Autodesk Inventor part; units mm, degrees
ref_plane "YZ Plane" through (0, 0, 0) normal (1, 0, 0) x (0, 1, 0)
ref_plane "XZ Plane" through (0, 0, 0) normal (0, 1, 0) x (-1, 0, 0)
ref_plane "XY Plane" through (0, 0, 0) normal (0, 0, 1) x (1, 0, 0)
sketch "Sketch1" plane through (0, 0, 0) normal (1, 0, 0) x (0, 1, 0)
  line L0 (0, 0) -> (-40.0558, 0)
  line L1 (-40.0558, 0) -> (-40.0558, -6.35)
  line L2 (-40.0558, -6.35) -> (0, -6.35)
  line L3 (0, -6.35) -> (0, 0)
  line L4 (-23.495, -6.35) -> (-34.0019, 4.1569)
  line L5 (-34.0019, 4.1569) -> (-42.2823, -4.1235)
  line L6 (-42.2823, -4.1235) -> (-31.7754, -14.6304)
  line L7 (-31.7754, -14.6304) -> (-23.495, -6.35)
  line L8 (-23.495, -6.35) -> (-8.636, -6.35) construction
  line L9 (-23.495, -6.35) -> (0, -6.35) construction
  dimension "d0" = 40.0558
  dimension "d2" = 6.35
  dimension "d3" = 14.859
  dimension "d4" = 135
  dimension "d6" = 23.495
extrude "Extrusion1" add sketch "Sketch1" along normal blind 26.3652
sketch "Sketch2" plane through (26.3652, 0, 0) normal (1, 0, 0) x (0, 0, -1)
  line L0 (6.35, -23.495) -> (6.35, 0)
  line L1 (6.35, 0) -> (0, 0)
  line L2 (0, 0) -> (0, -29.845)
  line L3 (14.6304, -31.7754) -> (6.35, -23.495)
  line L4 (6.35, -23.495) -> (0, -29.845)
  line L5 (0, -29.845) -> (0, 0)
  line L6 (0, 0) -> (6.35, 0)
  line L7 (6.35, 0) -> (6.35, -23.495)
extrude "Extrusion2" cut sketch "Sketch2" against normal blind 16.2052
sketch "Sketch5" plane through (0, 0, 0) normal (-1, 0, 0) x (0, 0, 1)
  line L0 (-4.1235, -42.2823) -> (-14.6304, -31.7754)
  line L1 (-6.35, -23.495) -> (-6.35, 0)
  line L2 (-6.35, -23.495) -> (-6.35, -40.0558)
  line L3 (-6.35, -40.0558) -> (-14.6304, -31.7754)
  line L4 (-14.6304, -31.7754) -> (-6.35, -23.495)
extrude "Extrusion5" cut sketch "Sketch5" against normal blind 12.7
sketch "Sketch6" plane through (26.3652, -23.495, -6.35) normal (0, 0.7071, -0.7071) x (-1, 0, 0)
  line L0 (13.6652, -11.7103) -> (0, -11.7103)
  circle A0 centre (6.8326, -5.8551) radius 4.5085
  line L1 (13.6652, 0) -> (0, 0)
  line L2 (0, -11.7103) -> (0, 0)
  line L3 (6.8326, -5.8551) -> (6.8326, 0) construction
  line L4 (6.8326, -5.8551) -> (6.8326, -11.7103) construction
  point P0 (26.3652, 21.1036)
  dimension "d24" = 9.017
extrude "Extrusion6" cut sketch "Sketch6" against normal blind 25.4
sketch "Sketch7" plane through (0, 0, 0) normal (-1, 0, 0) x (0, 0, 1)
  line L0 (-6.35, 0) -> (-6.35, -40.0558)
  line L1 (-6.35, 0) -> (0, 0)
  circle A0 centre (-7.62, -34.9758) radius 2.54
  line L2 (-7.62, -34.9758) -> (-6.35, -34.9758) construction
  line L3 (-6.35, -34.9758) -> (-6.35, -40.0558) construction
  line L4 (-6.35, 0) -> (-6.35, -5.08) construction
  line L5 (-6.35, -5.08) -> (-7.62, -5.08) construction
  circle A1 centre (-7.62, -5.08) radius 2.54
  dimension "d27" = 1.27
  dimension "d29" = 5.08
  dimension "d30" = 5.08
  dimension "d31" = 5.08
  dimension "d32" = 1.27
  dimension "d33" = 5.08
extrude "Extrusion7" add sketch "Sketch7" against normal blind 6.35
sketch "Sketch8" plane through (0, 0, 0) normal (-1, 0, 0) x (0, 0, 1)
  line L0 (0, -29.845) -> (4.1569, -34.0019)
  line L1 (0, 0) -> (0, -29.845)
  line L2 (4.1569, -34.0019) -> (-4.1235, -42.2823)
  line L3 (-6.35, -7.2797) -> (-6.35, -32.7761)
  line L4 (4.1569, -34.0019) -> (4.1569, -26.3819)
  line L5 (4.1569, -26.3819) -> (0, -22.225)
  line L6 (0, -22.225) -> (0, -29.845)
  line L7 (4.1569, -34.0019) -> (0, -29.845)
  dimension "d42" = 7.62
extrude "Extrusion8" add sketch "Sketch8" against normal blind 12.1412
ref_plane "Work Plane1" through (12.1412, -6.35, -6.35) normal (1, 0, 0) x (0, 0, -1)
sketch "Sketch9" plane through (12.1412, -6.35, -6.35) normal (1, 0, 0) x (0, 0, -1)
  line L0 (-10.5069, 6.35) -> (-10.5069, -29.5569)
  line L1 (-6.35, -25.4) -> (-10.5069, -29.5569)
  line L2 (-6.35, -25.4) -> (-6.35, 0)
  circle A0 centre (-8.4284, -20.4934) radius 1.5875
  line L3 (-6.35, -20.4934) -> (-10.5069, -20.4934) construction
  line L4 (-8.4284, -20.4934) -> (-8.4284, -27.4784) construction
  point P0 (-6.35, 6.35)
  dimension "d38" = 3.175
  dimension "d39" = 6.985
extrude "Extrusion9" add sketch "Sketch9" along normal blind 2.54
sketch "Sketch10" plane through (26.3652, 0, 0) normal (1, 0, 0) x (0, 0, -1)
  line L0 (0, -40.0558) -> (1.897, -40.0558)
  line L1 (14.6304, -31.7754) -> (6.35, -23.495)
  line L2 (0, -38.1254) -> (1.897, -40.0558)
  line L3 (1.897, -40.0558) -> (0, -40.0558)
  line L4 (0, -38.1254) -> (0, -40.0558)
  line L5 (0, -38.1254) -> (1.897, -40.0558)
  point P0 (0, 0)
  dimension "d43" = 0.5
extrude "Extrusion10" cut sketch "Sketch10" against normal blind 38.1
sketch "Sketch11" plane through (14.6812, -26.8434, 2.0784) normal (1, 0, 0) x (0, 0, -1)
  circle A0 centre (0, 0) radius 1.5875
  circle A1 centre (0, 0) radius 1.5875
  line L0 (-1.5875, 0) -> (1.5875, 0)
  line L1 (1.5875, 0) -> (1.5875, -2.159)
  line L2 (1.5875, -2.159) -> (-1.5875, -2.159)
  line L3 (-1.5875, -2.159) -> (-1.5875, 0)
  point P0 (2.0784, 26.8434)
  dimension "d46" = 2.159
extrude "Extrusion11" add sketch "Sketch11" along normal blind 2.54
sketch "Sketch14" plane through (12.1412, -6.35, -6.35) normal (1, 0, 0) x (0, 0, -1)
  line L0 (-6.8465, -10.2985) -> (-15.1263, -2.0187)
  line L1 (8.2804, -25.4254) -> (0, -17.145)
  line L2 (-15.1263, -2.0187) -> (-25.6332, -12.5256)
  line L3 (-25.6332, -12.5256) -> (-17.3534, -20.8054)
  line L4 (-17.3534, -20.8054) -> (-6.8465, -10.2985)
  point P0 (-6.35, 6.35)
  dimension "d60" = 11.7094
  dimension "d61" = 14.859
extrude "Extrusion14" add sketch "Sketch14" along normal blind 13.6652
sketch "Sketch15" plane through (12.1412, -6.35, -6.35) normal (-1, 0, 0) x (0, 0, 1)
  line L0 (6.8465, -10.2985) -> (15.1263, -2.0187)
  line L1 (25.6332, -12.5256) -> (17.3534, -20.8054)
  line L2 (15.1263, -2.0187) -> (25.6332, -12.5256)
  line L3 (25.6332, -12.5256) -> (17.3534, -20.8054)
  line L4 (6.8465, -10.2985) -> (17.3534, -20.8054)
  line L5 (6.8465, -10.2985) -> (15.1263, -2.0187)
  point P0 (6.35, 6.35)
extrude "Extrusion15" add sketch "Sketch15" along normal up to surface (12.1412 mm away)
sketch "Sketch17" plane through (0, 0, 0) normal (-1, 0, 0) x (0, 0, 1)
  line L0 (-1.897, -40.0558) -> (0, -38.1254)
  line L1 (4.1569, -26.3819) -> (0, -22.225)
  line L2 (0, 0) -> (0, -22.225)
  line L3 (-6.35, -37.1755) -> (-6.35, -40.0558)
  line L4 (-1.897, -40.0558) -> (-4.1235, -42.2823)
  line L5 (0, 0) -> (0, -22.225)
  line L6 (0, -22.225) -> (3.1163, -19.1087)
  line L7 (3.1163, -19.1087) -> (11.1874, -11.0376)
  line L8 (11.1874, -11.0376) -> (8.66, -8.5101)
  line L9 (8.66, -8.5101) -> (0, 0)
extrude "Extrusion17" add sketch "Sketch17" against normal up to surface (10.16 mm away)
sketch "Sketch18" plane through (25.8064, -8.3687, 8.7763) normal (0, 0.7071, -0.7071) x (-1, 0, 0)
  circle A0 centre (6.5407, -5.8547) radius 4.5085
  point P0 (25.8064, -0.2882)
  dimension "d70" = 9.017
extrude "Extrusion18" cut sketch "Sketch18" against normal up to surface (14.859 mm away)
sketch "Sketch19" plane through (26.3652, 0, 0) normal (1, 0, 0) x (0, 0, -1)
  line L0 (0, -38.1588) -> (0, -38.1254)
  line L1 (0, -38.1254) -> (1.897, -40.0558)
  line L2 (1.897, -40.0558) -> (4.1235, -42.2823)
  line L3 (14.6304, -31.7754) -> (6.35, -23.495)
  line L4 (-4.1569, -34.0019) -> (0, -38.1588)
  line L5 (-4.1569, -34.0019) -> (6.35, -23.495)
  line L6 (14.6304, -31.7754) -> (6.35, -23.495)
  line L7 (14.6304, -31.7754) -> (4.1235, -42.2823)
  line L8 (-4.1569, -34.0019) -> (4.1235, -42.2823)
  point P0 (0, 0)
extrude "Extrusion19" cut sketch "Sketch19" against normal up to surface (16.2052 mm away) contours L4 L5 L3 L7 L2 L1 L0
sketch "Sketch21" plane through (10.16, 0, 0) normal (1, 0, 0) x (0, 0, -1)
  line L0 (-8.6473, -8.4977) -> (0, 0)
  line L1 (0, 0) -> (-19.2606, -18.9274)
  line L2 (-19.2606, -18.9274) -> (-25.9368, -12.1336)
  line L3 (0, 0) -> (-6.6762, 6.7937)
  line L4 (-6.6762, 6.7937) -> (-25.9368, -12.1336)
  line L5 (0, 0) -> (-4.5719, 0)
  line L6 (-4.5719, 0) -> (-13.5895, 0)
  dimension "d75" = 9.525
extrude "Extrusion21" add sketch "Sketch21" against normal up to surface (10.16 mm away) contours L1 L2 L4 L6 L5 L0
sketch "Sketch22" plane through (10.16, 0, 0) normal (1, 0, 0) x (0, 0, -1)
  line L0 (-8.7763, -8.3687) -> (-19.2832, -18.8756)
  circle A0 centre (-18.8774, -12.1837) radius 1.588
  line L1 (-25.9368, -12.1336) -> (-19.2606, -18.9274)
  point P0 (0, 0)
  dimension "d81" = 3.176
  dimension "d82" = 4.445
  dimension "d95" = 5
extrude "Extrusion22" [suppressed]
sketch "Sketch23" plane through (24.2316, -12.1837, 18.8774) normal (1, 0, 0) x (0, 0, -1)
  circle A0 centre (0, 0) radius 1.588
  circle A1 centre (0, 0) radius 1.588
  line L0 (0.0027, 1.588) -> (-2.1563, 1.588)
  line L1 (-2.1563, 1.588) -> (-2.1563, -1.588)
  line L2 (-2.1563, -1.588) -> (0.0027, -1.588)
  line L3 (0.0027, -1.588) -> (0.0027, 1.588)
  point P0 (18.8774, 12.1837)
  dimension "d85" = 2.159
extrude "Extrusion23" [suppressed]
sketch "Sketch24" plane through (10.16, 0, 0) normal (1, 0, 0) x (0, 0, -1)
  line L0 (6.35, 0) -> (6.35, -40.0558)
  line L1 (-13.5895, 0) -> (6.35, 0)
  line L2 (-13.5895, 0) -> (-25.9368, -12.1336)
  line L3 (-25.9368, -12.1336) -> (-19.2606, -18.9274)
  line L4 (-19.2606, -18.9274) -> (-19.2459, -18.9129)
  line L5 (-19.2832, -18.8756) -> (-19.2459, -18.9129)
  line L6 (-8.7763, -8.3687) -> (-19.2832, -18.8756)
  line L7 (-0.4965, -16.6485) -> (-8.7763, -8.3687)
  line L8 (-3.0365, -19.1885) -> (-0.4965, -16.6485)
  line L9 (0, -22.225) -> (-3.0365, -19.1885)
  line L10 (0, -29.845) -> (0, -22.225)
  line L11 (-4.1569, -34.0019) -> (0, -29.845)
  line L12 (0, -38.1588) -> (-4.1569, -34.0019)
  line L13 (0, -38.1254) -> (0, -38.1588)
  line L14 (1.897, -40.0558) -> (0, -38.1254)
  line L15 (4.1235, -42.2823) -> (1.897, -40.0558)
  line L16 (6.35, -40.0558) -> (4.1235, -42.2823)
  line L17 (-4.1569, -34.0019) -> (0, -34.0019)
  line L18 (0, -34.0019) -> (0, -22.225)
  line L19 (0, -22.225) -> (-4.1569, -22.225)
  line L20 (-4.1569, -22.225) -> (-4.1569, -34.0019)
  point P0 (0, 0)
extrude "Extrusion24" cut sketch "Sketch24" along normal up to surface (7.0612 mm away) contours L20 L19 L10 L11 | L11 L18 L17
sketch "Sketch25" plane through (10.16, 0, 0) normal (1, 0, 0) x (0, 0, -1)
  line L0 (-4.1569, -34.0019) -> (-4.1569, -26.3819)
  line L1 (-4.1569, -34.0019) -> (-4.1569, -26.3819)
  line L2 (-4.1569, -26.3819) -> (0, -22.225)
  line L3 (0, -22.225) -> (-3.0365, -19.1885)
  line L4 (-4.1569, -34.0019) -> (-11.3495, -26.8093)
  line L5 (-11.3495, -26.8093) -> (-3.0365, -19.1885)
  point P0 (0, 0)
extrude "Extrusion25" add sketch "Sketch25" against normal up to surface (10.16 mm away)
sketch "Sketch26" plane through (10.16, 0, 0) normal (1, 0, 0) x (0, 0, -1)
  circle A0 centre (-18.8774, -12.1837) radius 1.588
  circle A1 centre (-18.8774, -12.1837) radius 2.54
  point P0 (0, 0)
  dimension "d92" = 5.08
extrude "Extrusion26" [suppressed]
sketch "Sketch27" plane through (10.16, 0, 0) normal (1, 0, 0) x (0, 0, -1)
  circle A0 centre (-18.8774, -12.1837) radius 1.588
  line L0 (-25.9368, -12.1336) -> (-19.2606, -18.9274)
  line L1 (-13.5895, 0) -> (-25.9368, -12.1336)
  point P0 (0, 0)
  dimension "d96" = 5
  dimension "d97" = 4.9837
hole "Hole1" at (10.16, -12.1837, 18.8774) direction (-1, 0, 0) diameter 2.1565 end through all
properties part number "ScrewMount"
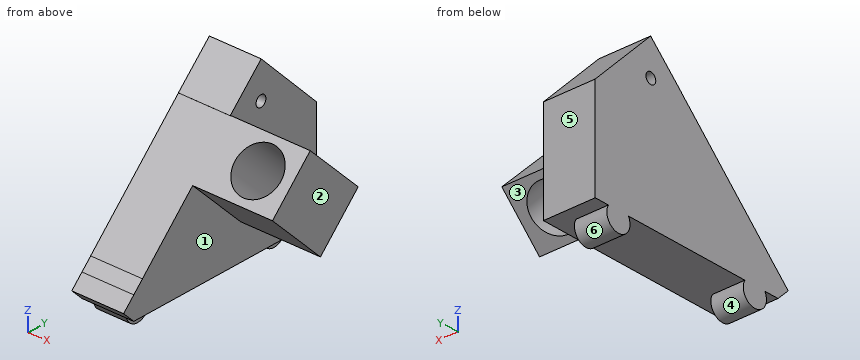
The model under review builds one solid part; all positions refer to its coordinate system, in mm. Face numbers are marked on the shaded views. A direction names the side the tool comes from. Give positions to 0.01 mm unless a question says otherwise; leave off trailing zeros. Write each loop counter-clockwise with the first axis right and the second up, starting at its lowest first coordinate (ties: lowest second). Pieces come first, ordered by that corner, then holes.
1. Tool access review of the marked faces 1 and 2: name each direction out of +Z, -Z, +X, -X, +Y, -Y from which nothing blocks a thin tool from reaching the whole face with its end or side.
2. Add section D-D, the plane y = -5.5. Write out the cut boundary in (x, z).
3. For P1, Ø12, axis at x = 7, z = 14.5, coming from the -Y side; P2, Ø1.9, axis at y = -5, z = -8, coming from the +X side; P3, Ø1, axis at x = 21.5, z = -0.5, coming from the +Y side; P4, Ø3.5, axis at y = -12.18, z = 18.88, coming from the +X side, all flat-tipped, find the tip position at first contact; note any pin that passes through.
4. Draft analysis for pull direction Z (two halves, no side actions). For the marked faces 3, 4, 5 and 6, state which applies: +Z half, -Z half, draft (parallel to the pull), parting line (faces both ways), or undercut.
5. Add section A-A, the plane x = 16.5. Write out the cut boundary in (y, z), plus the area to 3 significant figures.
6. Add section B-B, the plane z = -7.62. Write out the cut boundary in (x, y).
Worked answers:
1. face 1: +X
1. face 2: +Z, -Z, +X, +Y, -Y
2. outline: (0, -10.13) - (6.35, -10.13) - (6.35, -6.35) - (10.16, -6.35) - (10.16, 19.19) - (0, 19.19) - close
3. P1: stops at y = -29.66
3. P2: stops at x = 6.35
3. P3: passes through
3. P4: stops at x = 10.16
4. face 3: -Z half
4. face 4: undercut
4. face 5: draft
4. face 6: undercut
5. outline: (-27.16, 11) - (-16.65, 0.5) - (-15.03, 2.12) - (-25.53, 12.63) - close; (-20.5, 17.66) - (-9.99, 7.15) - (-8.37, 8.78) - (-18.88, 19.28) - close
5. area: 68.2 mm2
6. outline: (0, -37.52) - (6.35, -37.52) - (6.35, -32.44) - (0, -32.44) - close; (0, -7.62) - (6.35, -7.62) - (6.35, -2.54) - (0, -2.54) - close
